Build history of the part. All positions in model axes, mm. A direction names the side the tool comes from. Round coordinates to 2 decimals unless told otherwise and drop trailing zeros. Loops run counter-clockwise (first coordinate to the right, second up) from the corner with the lowest first, then second, coordinate; pieces in that order, holes last.
from build123d import *

# Parameters (mm, degrees)
BOSS_EXTRUDE1_DEPTH = 6.35
SKETCH2_R           = 3.302
CUT_EXTRUDE3_DEPTH  = 6.35


with BuildPart() as part:
    # Sketch1 → Boss-Extrude1 (new body)
    with BuildSketch(Plane.XY):
        with BuildLine():
            Line((914.4, 0), (838.2, 0))
            Line((838.2, 0), (838.2, -12.7))
            Line((838.2, -12.7), (965.2, -50.8))
            Line((965.2, -50.8), (971.677, -50.8))
            Line((971.677, -50.8), (971.677, -26.67))
            ThreePointArc((971.677, -26.67), (990.6635, -7.6835), (1009.65, -26.67))
            Line((1009.65, -26.67), (1009.65, -50.8))
            Line((1009.65, -50.8), (1016, -50.8))
            Line((1016, -50.8), (1016, 50.8))
            Line((1016, 50.8), (965.2, 50.8))
            Line((965.2, 50.8), (914.4, 50.8))
            Line((914.4, 50.8), (914.4, 0))
        make_face()
    extrude(amount=BOSS_EXTRUDE1_DEPTH)

    # Sketch2 → Cut-Extrude3 (cut)
    with BuildSketch(Plane.XY.offset(6.35)):
        with Locations((990.6, 25.4)):
            Circle(SKETCH2_R)
    extrude(amount=-CUT_EXTRUDE3_DEPTH, mode=Mode.SUBTRACT)


solid = part.part
(1) Slice it at B-B on z = 5. List the corners of the cut face in (x, y), plus the area to 3 significant figures.
Responses:
outline: (838.2, -12.7) - (965.2, -50.8) - (971.68, -50.8) - (971.68, -26.67) arc R18.99 cw to (1009.65, -26.67) - (1009.65, -50.8) - (1016, -50.8) - (1016, 50.8) - (914.4, 50.8) - (914.4, 0) - (838.2, 0) - close; hole circle Ø6.6 at (990.6, 25.4)
area: 10,300 mm2
(2) Slice it at D-D on x = 922.5. List the corners of the cut face in (y, z), plus the area to 3 significant figures.
Responses:
outline: (-37.99, 0) - (50.8, 0) - (50.8, 6.35) - (-37.99, 6.35) - close
area: 564 mm2
(3) Probe line 1 (Y direction, x = 990.6, z = 2.75); line 2 (X direction, y = 22.5, z = 3.5); line 3 (X direction, y = 36, z = 0.5). List the from-to ranges inside material, lowest first.
Responses:
line 1: y = -7.68 to 22.1, 28.7 to 50.8
line 2: x = 914.4 to 989.02, 992.18 to 1016
line 3: x = 914.4 to 1016
(4) Which spindle directions (+Z, -Z, +X, -X, +Y, -Y) get a long thin tool onto all of the face, cutting with end or side? Do faces 4 (the face through (987.3, 25.5, 3.2)), 5 (the face through (1009.65, -39, 3)). Say none if no direction does.
Responses:
face 4: +Z, -Z
face 5: +Z, -Z, -Y
(5) Slice it at C-C on x = 990.6. List the corners of the cut face in (y, z), plus the area to 3 significant figures.
Responses:
outline: (-7.68, 0) - (22.1, 0) - (22.1, 6.35) - (-7.68, 6.35) - close; (28.7, 0) - (50.8, 0) - (50.8, 6.35) - (28.7, 6.35) - close
area: 329 mm2
(6) Pull direction X, two halves, no side cores. Call faces 1 (the face through (990.25, -7.69, 3.13)), 2 (the face through (914.4, 26, 3)), 3 (the face through (877, 0, 3)): +X half, -X half, draft (parallel to the pull), parting line (faces both ways), or undercut.
Responses:
face 1: undercut
face 2: -X half
face 3: draft
(7) Slice it at A-A on y = 25.4. List the corners of the cut face in (x, z), plus the area to 3 significant figures.
Responses:
outline: (914.4, 0) - (987.3, 0) - (987.3, 6.35) - (914.4, 6.35) - close; (993.9, 0) - (1016, 0) - (1016, 6.35) - (993.9, 6.35) - close
area: 603 mm2
(8) Pin check, flat tips, straight feed: P1, Ø1.9, axis at y = 31.5, z = 4.5, coming from the -X side; P2, Ø3, axis at x = 878.5, z = 3, coming from the +Y side; P3, Ø3, axis at x = 891.5, z = 3, coming from the -Y side; P4, Ø1.5, axis at x = 982.5, y = -12, coming from the +Z side. Stop position of each tip, or through.
Responses:
P1: stops at x = 914.4
P2: stops at y = 0
P3: stops at y = -29.14
P4: passes through
